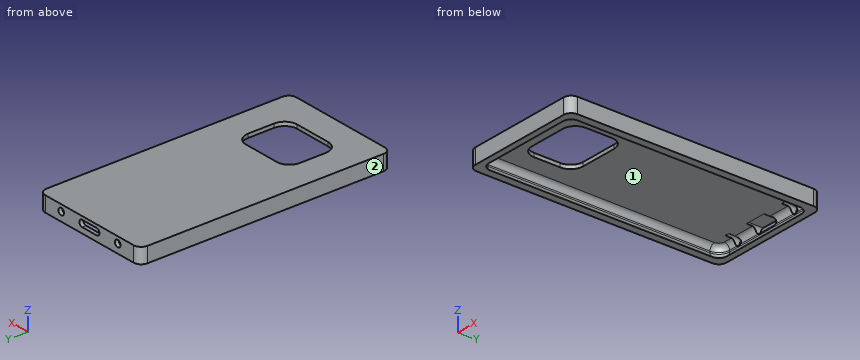
from build123d import *

# Parameters (mm, degrees)
EXTRUDE004_DEPTH = 10
SKETCH003_R      = 2.197673
EXTRUDE003_DEPTH = 10
EXTRUDE_DEPTH    = 8
FILLET_R         = 3.5
EXTRUDE001_DEPTH = 2.5
EXTRUDE002_DEPTH = 10


with BuildPart() as extrude004:
    # Sketch004 (on Face35 of Cut) → Extrude004 (new body)
    with BuildSketch(Plane(origin=(0, 0, 8), x_dir=(1, 0, 0), z_dir=(0, 0, -1))):
        with BuildLine():
            ThreePointArc((-12.218708, 64.166268), (-18.089957, 61.734317), (-20.521908, 55.863067))
            Line((-20.521908, 38.765661), (-20.521908, 55.863067))
            ThreePointArc((-20.521908, 38.765661), (-18.089957, 32.894412), (-12.218708, 30.462461))
            Line((12.218708, 30.462461), (-12.218708, 30.462461))
            ThreePointArc((12.218708, 30.462461), (18.089957, 32.894412), (20.521908, 38.765661))
            Line((20.521908, 55.863067), (20.521908, 38.765661))
            ThreePointArc((20.521908, 55.863067), (18.089957, 61.734317), (12.218708, 64.166268))
            Line((-12.218708, 64.166268), (12.218708, 64.166268))
        make_face()
    extrude(amount=-EXTRUDE004_DEPTH)


with BuildPart() as compound_features_to_remove:
    # Sketch003 (on Face6 of Cut) → Extrude003 (new body)
    with BuildSketch(Plane(origin=(0, 82.5, 0), x_dir=(-1, 0, 0), z_dir=(0, 1, 0))):
        with Locations((-22.370322, 6.27106)):
            Circle(SKETCH003_R)
        with Locations((22.370322, 6.27106)):
            Circle(SKETCH003_R)
        with BuildLine():
            ThreePointArc((5.787986, 4.150016), (7.90903, 6.27106), (5.787986, 8.392104))
            Line((5.787986, 8.392104), (-5.787986, 8.392104))
            ThreePointArc((-5.787986, 8.392104), (-7.90903, 6.27106), (-5.787986, 4.150016))
            Line((-5.787986, 4.150016), (5.787986, 4.150016))
        make_face()
    extrude(amount=-EXTRUDE003_DEPTH)

    # Compound: union Extrude004
    add(extrude004.part)


with BuildPart() as fillet_body:
    # Sketch → Extrude (new body)
    with BuildSketch(Plane.XY):
        with BuildLine():
            ThreePointArc((-29.5, 80), (-34.449747, 77.949747), (-36.5, 73))
            Line((-36.5, -73), (-36.5, 73))
            ThreePointArc((-36.5, -73), (-34.449747, -77.949747), (-29.5, -80))
            Line((29.5, -80), (-29.5, -80))
            ThreePointArc((29.5, -80), (34.449747, -77.949747), (36.5, -73))
            Line((36.5, 73), (36.5, -73))
            ThreePointArc((36.5, 73), (34.449747, 77.949747), (29.5, 80))
            Line((-29.5, 80), (29.5, 80))
        make_face()
    extrude(amount=EXTRUDE_DEPTH)

    # Fillet
    fillet_edges = [fillet_body.edges().sort_by_distance(p)[0] for p in [
        (-34.449747, 77.949747, 0),
        (-34.449747, 77.949747, 8),
        (-36.5, 0, 0),
        (-36.5, 0, 8),
        (-34.449747, -77.949747, 0),
        (-34.449747, -77.949747, 8),
        (0, -80, 0),
        (0, -80, 8),
        (34.449747, -77.949747, 0),
        (34.449747, -77.949747, 8),
        (36.5, 0, 0),
        (36.5, 0, 8),
        (34.449747, 77.949747, 0),
        (34.449747, 77.949747, 8),
        (0, 80, 0),
        (0, 80, 8),
    ]]
    fillet(fillet_edges, radius=FILLET_R)


with BuildPart() as obj1:
    # Sketch001 (on Face9 of Fillet) → Extrude001 (new body, symmetric)
    with BuildSketch(Plane(origin=(0, 0, 0), x_dir=(1, 0, 0), z_dir=(0, 0, -1))):
        with BuildLine():
            ThreePointArc((-29.5, 78.25), (-33.212311, 76.712311), (-34.75, 73))
            Line((-34.75, -73), (-34.75, 73))
            ThreePointArc((-34.75, -73), (-33.212311, -76.712311), (-29.5, -78.25))
            Line((29.5, -78.25), (-29.5, -78.25))
            ThreePointArc((29.5, -78.25), (33.212311, -76.712311), (34.75, -73))
            Line((34.75, 73), (34.75, -73))
            ThreePointArc((34.75, 73), (33.212311, 76.712311), (29.5, 78.25))
            Line((-29.5, 78.25), (29.5, 78.25))
        make_face()
    extrude(amount=EXTRUDE001_DEPTH, both=True)

    # Fusion: union Fillet body
    add(fillet_body.part)


with BuildPart() as cut001:
    # Sketch002 (on Face4 of Fusion) → Extrude002 (new body)
    with BuildSketch(Plane(origin=(0, 0, 0.5), x_dir=(1, 0, 0), z_dir=(0, 0, -1))):
        with BuildLine():
            Line((-35, 82.5), (35, 82.5))
            ThreePointArc((40, 77.5), (38.535534, 81.035534), (35, 82.5))
            Line((40, 77.5), (40, -77.5))
            ThreePointArc((35, -82.5), (38.535534, -81.035534), (40, -77.5))
            Line((35, -82.5), (-35, -82.5))
            ThreePointArc((-40, -77.5), (-38.535534, -81.035534), (-35, -82.5))
            Line((-40, -77.5), (-40, 77.5))
            ThreePointArc((-35, 82.5), (-38.535534, 81.035534), (-40, 77.5))
        make_face()
    extrude(amount=-EXTRUDE002_DEPTH)

    # Cut: cut obj1
    add(obj1.part, mode=Mode.SUBTRACT)

    # Cut001: cut  Compound - Features to remove
    add(compound_features_to_remove.part, mode=Mode.SUBTRACT)


solid = cut001.part
The listing builds one solid part. Answer for the finished solid, in the listing's coordinates (mm). Face numbers are marked on the shaded views. Coordinates: 2 decimals unless noted, no trailing zeros. Order: outer loops, then holes, each group sorted by start corner. A loop starts at its lowest first (then second) coordinate and runs counter-clockwise, first axis right, second up.
Q1. A cutting plane is placed at D-D, the plane x = 16.5. Write down the section's boundary in (y, z), and give its area (3 significant figures).
Q2. Given P1, Ø2, axis at x = 13.5, y = -2.5, coming from the -Z side; P2, Ø2.5, axis at x = 22.37, z = 6.27, coming from the +Y side; P3, Ø1, axis at x = -4.5, z = 6, coming from the +Y side, each flat-ended and moving along its own axis, determine where each tip first touches the part or whether it passes through.
Q3. A cutting plane is placed at C-C, the plane y = -32. Write down the section's boundary in (x, z), and give its area (3 significant figures).
Q4. A cutting plane is placed at B-B, the plane y = 16. Write down the section's boundary in (x, z).
Q5. Consider line 1 (Y direction, x = -2, z = 3.5); line 2 (X direction, y = -56, z = 3.75); line 3 (Y direction, x = 26, z = 7.5). Determine where each line is inside the solid, lowest interval first.
Q6. A cutting plane is placed at A-A, the plane x = -3. Write down the section's boundary in (y, z).
Q7. For a pull along Y with two mould halves and no side action, classify the marked faces 1 and 2 as pulls with the +Y half, pulls with the -Y half, needs draft (parallel to the pull), parting line crosses it, or undercut.
Answers follow:
1. outline: (-82.5, 0.5) - (-78.3, 0.5) arc R3.5 cw to (-80, 3.5) - (-80, 4.5) arc R3.5 cw to (-76.5, 8) - (-62.98, 8) - (-62.98, 10.5) - (-82.5, 10.5) - close; (-31.65, 8) - (76.5, 8) arc R3.5 cw to (80, 4.5) - (80, 3.5) arc R3.5 cw to (78.3, 0.5) - (82.5, 0.5) - (82.5, 10.5) - (-31.65, 10.5) - close
1. area: 380 mm2
2. P1: stops at z = 8
2. P2: stops at y = -78.27
2. P3: stops at y = -79.37
3. outline: (-40, 0.5) - (-34.8, 0.5) arc R3.5 cw to (-36.5, 3.5) - (-36.5, 4.5) arc R3.5 cw to (-33, 8) - (-17.03, 8) - (-17.03, 10.5) - (-40, 10.5) - close; (17.03, 8) - (33, 8) arc R3.5 cw to (36.5, 4.5) - (36.5, 3.5) arc R3.5 cw to (34.8, 0.5) - (40, 0.5) - (40, 10.5) - (17.03, 10.5) - close
3. area: 176 mm2
4. outline: (-40, 0.5) - (-34.8, 0.5) arc R3.5 cw to (-36.5, 3.5) - (-36.5, 4.5) arc R3.5 cw to (-33, 8) - (33, 8) arc R3.5 cw to (36.5, 4.5) - (36.5, 3.5) arc R3.5 cw to (34.8, 0.5) - (40, 0.5) - (40, 10.5) - (-40, 10.5) - close
5. line 1: y = -82.5 to -80, 80 to 82.5
5. line 2: x = -40 to -36.5, 36.5 to 40
5. line 3: y = -82.5 to -78.3, 78.3 to 82.5
6. outline: (-82.5, 0.5) - (-78.3, 0.5) arc R3.5 cw to (-80, 3.5) - (-80, 4.5) arc R3.5 cw to (-76.5, 8) - (-64.17, 8) - (-64.17, 10.5) - (-82.5, 10.5) - close; (-30.46, 8) - (72.5, 8) - (72.5, 8.39) - (82.5, 8.39) - (82.5, 10.5) - (-30.46, 10.5) - close; (78.3, 0.5) - (82.5, 0.5) - (82.5, 4.15) - (80, 4.15) - (80, 3.5) arc R3.5 cw to start
7. face 1: undercut
7. face 2: needs draft
